Check sheet for the modelled part. Datum: model origin and axes. Units: mm. Face numbers are marked on the shaded views. Round coordinates to 2 decimals unless told otherwise and drop trailing zeros. Write each loop counter-clockwise with the first axis right and the second up, starting at its lowest first coordinate (ties: lowest second). Pieces come first, ordered by that corner, then holes. Notation, with made-up numbers: (86.5, 16) - (118.5, 16) arc R22 ccw to (118.5, 37) - close; hole circle Ø3 at (61, -4.75). An arc over 180 degrees is marked (long way). Use one line per item in the form item = value. Start each with the question number.
1) Draft check along Y on the marked faces 1, 2, 3 and 4. Enter one of: +Y half, -Y half, draft (parallel to the pull), parting line (faces both ways), or undercut.
2) Section check D-D (z = 20). Record the boundary of the cut face in (x, y), then the cut area to 3 significant figures.
3) Section check A-A (z = 43.5). Record the boundary of the cut face in (x, y).
4) Scan lines: probe 1 along Z at (x, y) = (-63, 109.25); probe 2 along Y at (x, z) = (-58.55, 20); probe 3 along Y at (x, z) = (-61, 48). Record each from-to range of solid material in increasing order.
5) Section check B-B (x = -59.75). Record the boundary of the cut face in (y, z).
6) Section check C-C (y = 116.75). Record the boundary of the cut face in (x, z).
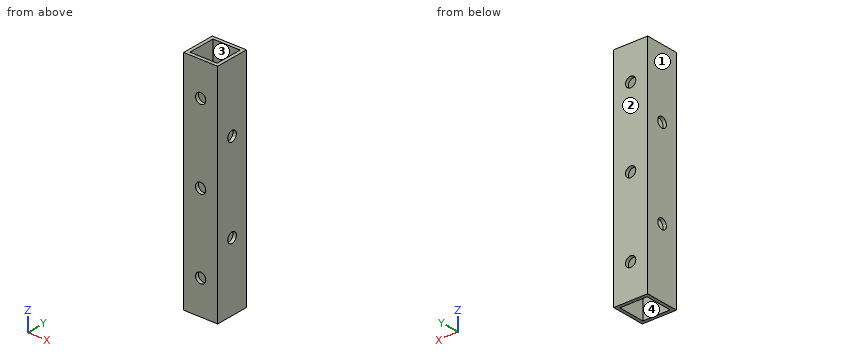
from build123d import *

# Parameters (mm, degrees)
SKETCH_1_W          = 10
SKETCH_1_H          = 10
SKETCH_1_W_2        = 8
SKETCH_1_H_2        = 8
EXTRUDE_1_DEPTH     = 66
SKETCH_2_R          = 1.5
CUT_EXTRUDE_1_DEPTH = 11
SKETCH_3_R          = 1.5
CUT_EXTRUDE_2_DEPTH = 11


with BuildPart() as part:
    # 草图1 → 拉伸-薄壁1 (new body)
    with BuildSketch(Plane.XY):
        with Locations((-63.129584871, 113.346996024)):
            Rectangle(SKETCH_1_W, SKETCH_1_H)
        with Locations((-63.129584871, 113.346996024)):
            Rectangle(SKETCH_1_W_2, SKETCH_1_H_2, mode=Mode.SUBTRACT)
    extrude(amount=EXTRUDE_1_DEPTH)

    # 草图2 → 切除-拉伸1 (cut, through all)
    with BuildSketch(Plane(origin=(-58.129584871, 0, 0), x_dir=(0, 0, -1), z_dir=(1, 0, 0))):
        with Locations((-20, 113.346996024)):
            Circle(SKETCH_2_R)
        with Locations((-46, 113.346996024)):
            Circle(SKETCH_2_R)
    extrude(amount=-CUT_EXTRUDE_1_DEPTH, mode=Mode.SUBTRACT)

    # 草图3 → 切除-拉伸2 (cut, through all)
    with BuildSketch(Plane.XZ.offset(-108.346996024)):
        with Locations((-63.129584871, 10)):
            Circle(SKETCH_3_R)
        with Locations((-63.129584871, 56)):
            Circle(SKETCH_3_R)
        with Locations((-63.129584871, 33)):
            Circle(SKETCH_3_R)
    extrude(amount=-CUT_EXTRUDE_2_DEPTH, mode=Mode.SUBTRACT)


solid = part.part
Results are:
q1.face_1 = draft
q1.face_2 = +Y half
q1.face_3 = undercut
q1.face_4 = undercut
q2.outline = (-68.13, 108.35) - (-58.13, 108.35) - (-58.13, 111.85) - (-59.13, 111.85) - (-59.13, 109.35) - (-67.13, 109.35) - (-67.13, 111.85) - (-68.13, 111.85) - close; (-68.13, 114.85) - (-67.13, 114.85) - (-67.13, 117.35) - (-59.13, 117.35) - (-59.13, 114.85) - (-58.13, 114.85) - (-58.13, 118.35) - (-68.13, 118.35) - close
q2.area = 30.0 mm²
q3.outline = (-68.13, 108.35) - (-58.13, 108.35) - (-58.13, 118.35) - (-68.13, 118.35) - close; hole (-67.13, 109.35) - (-59.13, 109.35) - (-59.13, 117.35) - (-67.13, 117.35) - close
q4.probe_1 = 0 to 8.51, 11.49 to 31.51, 34.49 to 54.51, 57.49 to 66
q4.probe_2 = 108.35 to 111.85, 114.85 to 118.35
q4.probe_3 = 108.35 to 109.35, 117.35 to 118.35
q5.outline = (108.35, 0) - (109.35, 0) - (109.35, 66) - (108.35, 66) - close; (117.35, 0) - (118.35, 0) - (118.35, 66) - (117.35, 66) - close
q6.outline = (-68.13, 0) - (-67.13, 0) - (-67.13, 66) - (-68.13, 66) - close; (-59.13, 0) - (-58.13, 0) - (-58.13, 66) - (-59.13, 66) - close
